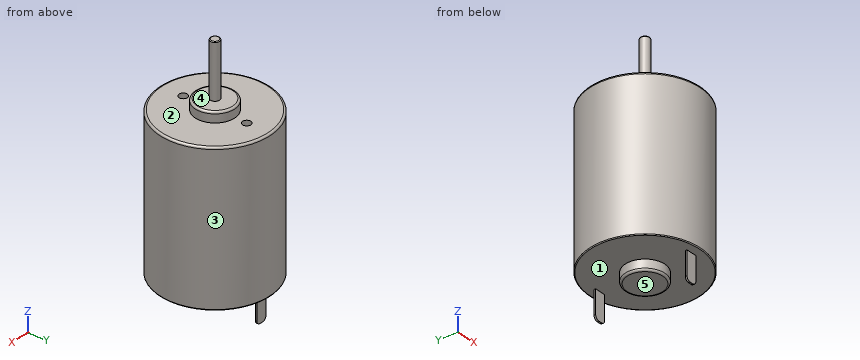
Autodesk Inventor part; units mm, degrees
ref_plane "YZ Plane" through (0, 0, 0) normal (1, 0, 0) x (0, 1, 0)
ref_plane "XZ Plane" through (0, 0, 0) normal (0, 1, 0) x (-1, 0, 0)
ref_plane "XY Plane" through (0, 0, 0) normal (0, 0, 1) x (1, 0, 0)
sketch "スケッチ1" plane through (0, 0, 0) normal (0, 0, 1) x (1, 0, 0)
  circle A0 centre (0, 0) radius 14
  dimension "d0" = 28
extrude "押し出し1" add sketch "スケッチ1" along normal blind 37.8
sketch "スケッチ2" plane through (0, 0, 37.8) normal (0, 0, 1) x (1, 0, 0)
  circle A0 centre (0, 0) radius 5
  dimension "d3" = 10
extrude "押し出し2" add sketch "スケッチ2" along normal blind 2.6
sketch "スケッチ3" plane through (0, 0, 40.4) normal (0, 0, 1) x (1, 0, 0)
  circle A0 centre (0, 0) radius 1.15
  dimension "d6" = 2.3
extrude "押し出し3" add sketch "スケッチ3" along normal blind 13.8
sketch "スケッチ4" plane through (0, 0, 0) normal (0, 0, -1) x (-1, 0, 0)
  circle A0 centre (0, 0) radius 1.15
  circle A1 centre (0, 0) radius 5
  dimension "d9" = 10
extrude "押し出し4" add sketch "スケッチ4" along normal blind 2.6 contours A0 | A1
sketch "スケッチ5" plane through (0, 0, 0) normal (0, 0, -1) x (-1, 0, 0)
  line L0 (1.4, -11.7) -> (-1.4, -11.7)
  line L1 (-1.4, -11.7) -> (-1.4, -11.3)
  line L2 (-1.4, -11.3) -> (1.4, -11.3)
  line L3 (1.4, -11.3) -> (1.4, -11.7)
  line L4 (1.4, 11.3) -> (-1.4, 11.3)
  line L5 (-1.4, 11.3) -> (-1.4, 11.7)
  line L6 (-1.4, 11.7) -> (1.4, 11.7)
  line L7 (1.4, 11.7) -> (1.4, 11.3)
  line L8 (0, 0) -> (0, -11.3)
  circle A0 centre (0, 0) radius 1.15
  line L9 (0, 0) -> (0, 11.3)
  dimension "d12" = 2.8
  dimension "d13" = 0.4
  dimension "d14" = 22.6
  dimension "d15" = 1.4
extrude "押し出し5" add sketch "スケッチ5" along normal blind 7 contours L4 L5 L6 L7 | L0 L1 L2 L3
fillet "フィレット1" radius 0.5 1 edges at (-14, 0, 37.8)
fillet "フィレット2" radius 0.2 1 edges at (-1.15, 0, 54.2)
fillet "フィレット3" radius 0.5 1 edges at (-5, 0, 40.4)
fillet "フィレット4" radius 0.5 1 edges at (5, 0, -2.6)
fillet "フィレット5" radius 1 1 edges at (-1.4, -11.5, -7)
fillet "フィレット6" radius 1 1 edges at (1.4, -11.5, -7)
fillet "フィレット7" radius 1 1 edges at (-1.4, 11.5, -7)
fillet "フィレット8" radius 1 1 edges at (1.4, 11.5, -7)
fillet "フィレット9" radius 0.2 1 edges at (-14, 0, 0)
sketch "スケッチ6" plane through (0, 0, 37.8) normal (0, 0, 1) x (1, 0, 0)
  circle A0 centre (0, 0) radius 8
  point P0 (0, 8)
  point P1 (0, -8)
  dimension "d27" = 16
hole "穴1" at (0, 8, 37.8) at (0, -8, 37.8) direction (0, 0, -1) diameter 2.113 depth 3
properties part number "RS-380"
Verification items for the finished model (mm, model axes). Face numbers are marked on the shaded views. A direction names the side the tool comes from. Give positions to 0.01 mm unless a question says otherwise; leave off trailing zeros. Write each loop counter-clockwise with the first axis right and the second up, starting at its lowest first coordinate (ties: lowest second). Pieces come first, ordered by that corner, then holes. Notation, with made-up numbers: (-25.5, -17.5) - (-2.5, -17.5) arc R14 cw to (-2.5, -8.5) - close; hole circle Ø3 at (19, 21.25). An arc over 180 degrees is marked (long way). Answer as CSV lines item,"result". Start each with the question number.
1. Draft check along Y on the marked faces 3, 4 and 5. Enter one of: pulls with the +Y half, pulls with the -Y half, needs draft (parallel to the pull), parting line crosses it, or undercut.
2. Thickness scan on line 1 (Y direction, x = 0, z = 36.6); line 2 (Z direction, x = 2, y = -12.25); line 3 (Z direction, x = -0.25, y = 8). Record the ranges inside material, lowest first.
3. Sectioned sample at B-B (y = 0). Record the boundary of the cut face in (x, z).
4. Sectioned sample at A-A (z = -1). Record the boundary of the cut face in (x, y), then the cut area to 3 significant figures.
5. Depth check by flat-ended pin: pin 1 (0.8 mm diameter, centred on x = -0.5, z = -5, fed in from +Y); pin 2 (1.3 mm diameter, centred on x = 0, y = 8, fed in from -Z); pin 3 (3 mm diameter, centred on x = 0.5, z = -3.5, fed in from -Y); pin 4 (5 mm diameter, centred on x = -9, z = 43, fed in from -Y). Enter the tip coordinate at first touch or a pass-through.
6. Sectioned sample at C-C (z = 31.5). Record the boundary of the cut face in (x, y).
7. Set-up check for the marked faces 1 and 2: record each of +Z, -Z, +X, -X, +Y, -Y from which the full face is reachable in a straight line by a thin tool's end or side.
Derived:
1,face 3,"parting line crosses it"
1,face 4,"needs draft"
1,face 5,"undercut"
2,line 1,"-14 to -9.06, -6.94 to 6.94, 9.06 to 14"
2,line 2,"0 to 37.8"
2,line 3,"0 to 34.8"
3,outline,"(-14, 0.2) arc R0.2 ccw to (-13.8, 0) - (-5, 0) - (-5, -2.1) arc R0.5 ccw to (-4.5, -2.6) - (4.5, -2.6) arc R0.5 ccw to (5, -2.1) - (5, 0) - (13.8, 0) arc R0.2 ccw to (14, 0.2) - (14, 37.3) arc R0.5 ccw to (13.5, 37.8) - (5, 37.8) - (5, 39.9) arc R0.5 ccw to (4.5, 40.4) - (1.15, 40.4) - (1.15, 54) arc R0.2 ccw to (0.95, 54.2) - (-0.95, 54.2) arc R0.2 ccw to (-1.15, 54) - (-1.15, 40.4) - (-4.5, 40.4) arc R0.5 ccw to (-5, 39.9) - (-5, 37.8) - (-13.5, 37.8) arc R0.5 ccw to (-14, 37.3) - close"
4,outline,"circle Ø10 at (0, 0); (-1.4, -11.7) - (1.4, -11.7) - (1.4, -11.3) - (-1.4, -11.3) - close; (-1.4, 11.3) - (1.4, 11.3) - (1.4, 11.7) - (-1.4, 11.7) - close"
4,area,"80.8 mm²"
5,pin 1,"y = 11.7"
5,pin 2,"z = 0"
5,pin 3,"y = -11.7"
5,pin 4,"through"
6,outline,"circle Ø28 at (0, 0)"
7,face 1,"-Z"
7,face 2,"+Z"
